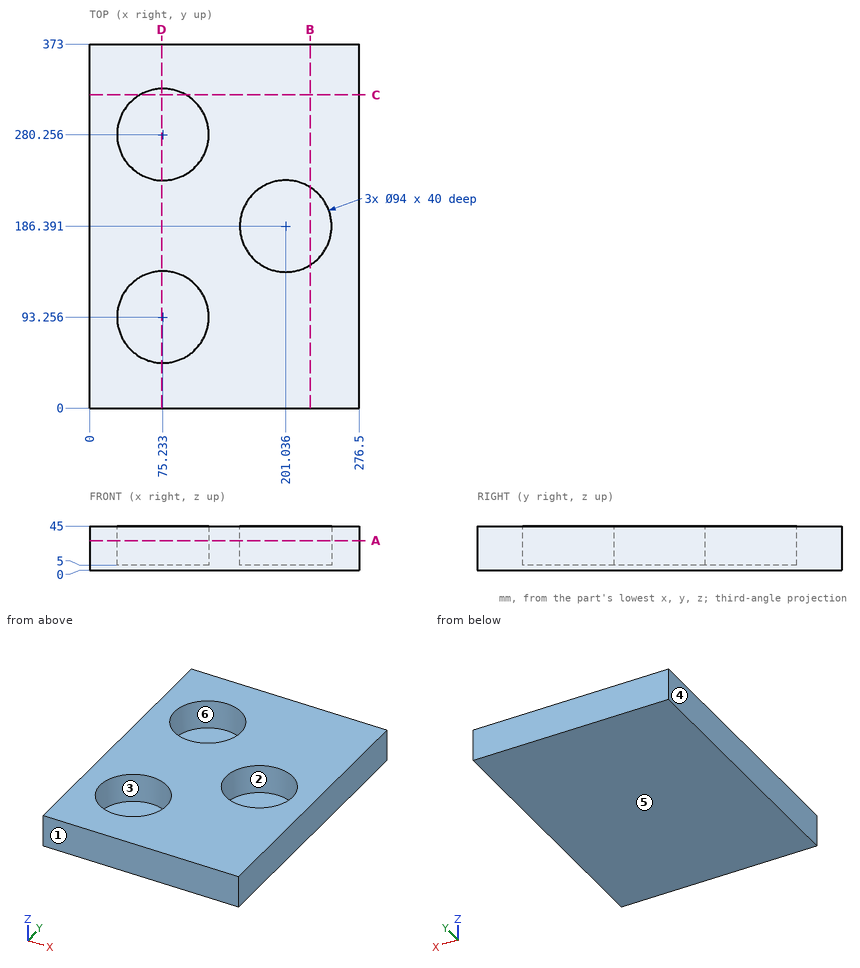
The drawing under review shows one solid part. Ordinate dimensions are in mm from its lowest x, y, z. A direction names the side the tool comes from. Coordinates: 2 decimals unless noted, no trailing zeros. Loops run counter-clockwise (first coordinate to the right, second up) from the corner with the lowest first, then second, coordinate; pieces in that order, holes last.
Item 1: Wall thickness on L1, parallel to Y at x = 67.5, z = 40 (1 decimal); L2, parallel to Y at x = 88, z = 18; L3, parallel to Y at x = 201.5, z = 6: over which ranges is each line inside the solid? List them lowest first.
Completed:
L1: y = 0 to 46.9, 139.6 to 233.9, 326.6 to 373
L2: y = 0 to 48.02, 138.49 to 235.02, 325.49 to 373
L3: y = 0 to 139.39, 233.39 to 373
Item 2: Add section A-A (z = 30). Write out the cut boundary in (x, y), and give its area (3 significant figures).
Completed:
outline: (0, 0) - (276.5, 0) - (276.5, 373) - (0, 373) - close; hole circle Ø94 at (75.23, 93.26); hole circle Ø94 at (75.23, 280.26); hole circle Ø94 at (201.04, 186.39)
area: 82,300 mm2
Item 3: Add section C-C (y = 321). Write out the cut boundary in (x, z), and give its area (3 significant figures).
Completed:
outline: (0, 0) - (276.5, 0) - (276.5, 45) - (98.66, 45) - (98.66, 5) - (51.8, 5) - (51.8, 45) - (0, 45) - close
area: 10,600 mm2
Item 4: Clearance check with flat-ended pins moving along their axes: pin 1 (1.5 mm diameter, centred on x = 178.5, z = 16, fed in from -Y); pin 2 (1 mm diameter, centred on x = 34, y = 78, fed in from +Z). State where each tip first meets the part, or that it passes through.
Completed:
pin 1: stops at y = 0
pin 2: stops at z = 5
Item 5: For the marked faces 5 and 6, list the 3-axis set-ups (+Z, -Z, +X, -X, +Y, -Y) from which the entire face can be reached by the end or side of a thin tool; tool diameter is ignored.
Completed:
face 5: -Z, +X, -X, +Y, -Y
face 6: +Z
Item 6: Add section B-B (x = 226). Write out the cut boundary in (y, z).
Completed:
outline: (0, 0) - (373, 0) - (373, 45) - (226.21, 45) - (226.21, 5) - (146.57, 5) - (146.57, 45) - (0, 45) - close
Item 7: Add section D-D (x = 74). Write out the cut boundary in (y, z).
Completed:
outline: (0, 0) - (373, 0) - (373, 45) - (327.24, 45) - (327.24, 5) - (233.27, 5) - (233.27, 45) - (140.24, 45) - (140.24, 5) - (46.27, 5) - (46.27, 45) - (0, 45) - close
Item 8: Draft analysis for pull direction Y (two halves, no side actions). For the marked faces 1, 2, 3 and 4, state which applies: pulls with the +Y half, pulls with the -Y half, needs draft (parallel to the pull), parting line crosses it, or undercut.
Completed:
face 1: pulls with the -Y half
face 2: undercut
face 3: undercut
face 4: needs draft
